```python
from build123d import *

# Parameters (mm, degrees)
SKETCH2_W     = 4
SKETCH2_H     = 3
CHAMFER1_SIZE = 3


with BuildPart() as part:
    # Sketch2 → Revolve1 (revolve)
    with BuildSketch(Plane.XY, mode=Mode.PRIVATE) as revolve1_sk:
        Polygon((-28, 0), (-3, 0), (-3, 8), (-7, 8), (-7, 12.96), (-28, 39), (-28, 36), (-28, 3), align=None)
        with Locations((-30, 1.5)):
            Rectangle(SKETCH2_W, SKETCH2_H)
        with Locations((-30, 37.5)):
            Rectangle(SKETCH2_W, SKETCH2_H)
    revolve(revolve1_sk.sketch.rotate(Axis((0, 0, 0), (0, 1, 0)), 270), axis=Axis((0, 0, 0), (0, 1, 0)))

    # Chamfer1
    chamfer1_edges = [part.edges().sort_by_distance(p)[0] for p in [
        (0, 39, 32),
    ]]
    chamfer(chamfer1_edges, length=CHAMFER1_SIZE - 0.0001)  # a hair under: the kernel refuses the full size


solid = part.part
```
CAD build for the part. Positions are in the model's coordinates, mm. A direction names the side the tool comes from. Round coordinates to 2 decimals unless told otherwise and drop trailing zeros. Order: outer loops, then holes, each group sorted by start corner. A loop starts at its lowest first (then second) coordinate and runs counter-clockwise, first axis right, second up.
Q1. Slice it at C-C (y = 6). Write the cut outline in (x, z), and give its area (3 significant figures).
Q2. Wall check: L1, parallel to X at y = 9.3, z = 0; L2, parallel to X at y = 6, z = 0; L3, parallel to Y at x = -14, z = -26. Give the ranges that are in metal, low to high.
Q3. Two-plate mould, pull along Y, no slides. Class faces 4 (the cylindrical face through (27.334, 19.269, 6.07)), 5 (the cylindrical face through (6.834, 10.515, 1.517)), 6 (the flat face through (28.3, 3, 0.1)), 7 (the conical face through (10.39, 17.48, 2.31)): pulls with the +Y half, pulls with the -Y half, needs draft (parallel to the pull), parting line crosses it, or undercut.
Q4. Drop flat-ended pins along their axis: pin 1 (1.5 mm diameter, centred on y = 13, z = -24, fed in from -X); pin 2 (19 mm diameter, centred on x = 12, z = 9.5, fed in from -Y); pin 3 (1 mm diameter, centred on x = 22.5, y = 14, fed in from +Z); pin 4 (10 mm diameter, centred on y = 11.5, z = -6, fed in from -X). Give the stop position or say it passes through.
Q5. Which spindle directions (+Z, -Z, +X, -X, +Y, -Y) get a long thin tool onto all of the face, cutting with end or side? Do faces 1 (the flat face through (3, 8, 1)), 2 (the cylindrical face through (31.24, 1.52, 6.94)), 3 (the flat face through (28.3, 36, 0.1)). Say none if no direction does.
Q6. Slice it at D-D (y = 15). Write the cut outline in (x, z).
Results below:
1. outline: circle Ø56 at (0, 0); hole circle Ø6 at (0, 0)
1. area: 2,430 mm2
2. L1: x = -28 to -7, 7 to 28
2. L2: x = -28 to -3, 3 to 28
2. L3: y = 0 to 3, 36 to 38.47
3. face 4: undercut
3. face 5: needs draft
3. face 6: undercut
3. face 7: pulls with the +Y half
4. pin 1: stops at x = -15.6
4. pin 2: stops at y = 0
4. pin 3: stops at z = 17.32
4. pin 4: stops at x = -27.98
5. face 1: +Y
5. face 2: +Y, -Y
5. face 3: none
6. outline: circle Ø56 at (0, 0); hole circle Ø17.29 at (0, 0)
